Read the model definition and answer for the solid it produces. Units are mm, in the model's axes. A direction names the side the tool comes from. Coordinates: 2 decimals unless noted, no trailing zeros. Order: outer loops, then holes, each group sorted by start corner. A loop starts at its lowest first (then second) coordinate and runs counter-clockwise, first axis right, second up. Notation, with made-up numbers: (-19, 10) -> (36, 10) arc R17 ccw to (36, 38) -> close; hole circle Ø1 at (-33.75, 33). An arc over 180 degrees is marked (long way). Answer as a JSON object with one key per item and string values. Group by question number.
1) A tool of negligible diameter and unlimited length cuts with its end or side. For faces 1 (the flat face through (-1, -1, -2)), 2 (the flat face through (18, 33, 128)), 3 (the flat face through (95, -4, -120)), 4 (the flat face through (100.08, -9.04, -1.68)), from which of +Z, -Z, +X, -X, +Y, -Y can it reach the whole face along a straight path? Write none if from no direction.
2) Section D-D on z = -28.5 is taken. Determine the outline of the cut face in (x, y).
3) Consider L1, parallel to X at y = -0.4, z = -52; L2, parallel to Y at x = -5.5, z = 36; L3, parallel to Z at x = -0.5, y = 13.5. Determine where each line is inside the solid, lowest interval first.
4) Section B-B on x = 0 is taken. Determine the outline of the cut face in (y, z).
5) Section C-C on y = 63.5 is taken. Determine the outline of the cut face in (x, z).
6) Given pin 1 (9 mm diameter, centred on x = 93.5, y = -6, fed in from +Z); pin 2 (19.5 mm diameter, centred on y = -12.5, z = -134, fed in from +X); pin 3 (1 mm diameter, centred on y = 0, z = -43.5, fed in from +X), each flat-ended and moving along its own axis, determine where each tip first touches the part or whether it passes through.
7) Determine the mould class of faces 5 (the flat face through (95, -4, 120)), 6 (the flat face through (-95.674, -3.727, 1.68)), 7 (the flat face through (-95, -4, -120)), 8 (the cylindrical face through (0.88, -0.49, -114.98)) for opening direction Z: released by +Z, released by -Z, zero draft, split by the parting line, or undercut.
8) Section A-A on z = -111 is taken. Determine the outline of the cut face in (x, y), and give its area (3 significant figures).
from build123d import *

# Parameters (mm, degrees)
ESBO_O1_W                 = 180
ESBO_O1_H                 = 250
FLANGE_BASE1_DEPTH        = 1
ESBO_O6_R                 = 2.4
ESBO_O6_R_2               = 20
CORTE_EXTRUS_O1_DEPTH     = 10
FILETE1_R                 = 5
ARESTA_FLANGE1_DEPTH      = 170
ARESTA_FLANGE2_DEPTH      = 240
ARESTA_FLANGE2_BEND_DEPTH = 240
FILETE2_R                 = 5
ARESTA_FLANGE3_DEPTH      = 170
FILETE3_R                 = 70
ESBO_O29_W                = 23
ESBO_O29_H                = 57
CORTE_EXTRUS_O2_DEPTH     = 308.427518565
FILETE4_R                 = 2
CORTE_EXTRUS_O3_REACH     = 220.213
ESBO_O32_R                = 2.4


# Sheet-metal steps are written as plain solids
with BuildPart() as part:
    # Esbo_o1 → Flange-base1 (new body)
    with BuildSketch(Plane(origin=(0, 0, 0), x_dir=(1, 0, 0), z_dir=(0, 1, 0))):
        Rectangle(ESBO_O1_W, ESBO_O1_H)
    extrude(amount=-FLANGE_BASE1_DEPTH)

    # Esbo_o6 → Corte-extrus_o1 (cut)
    with BuildSketch(Plane(origin=(0, 0, 0), x_dir=(1, 0, 0), z_dir=(0, 1, 0))):
        with Locations(Location((-25, 52, 0), (0, 0, 270))):
            Circle(ESBO_O6_R)
        with Locations(Location((25, 52, 0), (0, 0, 270))):
            Circle(ESBO_O6_R)
        with Locations(Location((-25, -40, 0), (0, 0, 270))):
            Circle(ESBO_O6_R)
        with Locations(Location((25, -40, 0), (0, 0, 270))):
            Circle(ESBO_O6_R)
        with Locations(Location((-25, -46, 0), (0, 0, 270))):
            Circle(ESBO_O6_R)
        with Locations(Location((25, -46, 0), (0, 0, 270))):
            Circle(ESBO_O6_R)
        with Locations(Location((-25, 46, 0), (0, 0, 270))):
            Circle(ESBO_O6_R)
        with Locations(Location((25, 46, 0), (0, 0, 270))):
            Circle(ESBO_O6_R)
        with Locations(Location((-25, 58, 0), (0, 0, 270))):
            Circle(ESBO_O6_R)
        with Locations(Location((25, 58, 0), (0, 0, 270))):
            Circle(ESBO_O6_R)
        with Locations(Location((-25, -34, 0), (0, 0, 270))):
            Circle(ESBO_O6_R)
        with Locations(Location((25, -34, 0), (0, 0, 270))):
            Circle(ESBO_O6_R)
        with Locations(Location((-25, 40, 0), (0, 0, 270))):
            Circle(ESBO_O6_R)
        with Locations(Location((25, 40, 0), (0, 0, 270))):
            Circle(ESBO_O6_R)
        with Locations(Location((-25, -52, 0), (0, 0, 270))):
            Circle(ESBO_O6_R)
        with Locations(Location((25, -52, 0), (0, 0, 270))):
            Circle(ESBO_O6_R)
        with Locations(Location((-25, 34, 0), (0, 0, 270))):
            Circle(ESBO_O6_R)
        with Locations(Location((25, 34, 0), (0, 0, 270))):
            Circle(ESBO_O6_R)
        with Locations(Location((-25, -58, 0), (0, 0, 270))):
            Circle(ESBO_O6_R)
        with Locations(Location((25, -58, 0), (0, 0, 270))):
            Circle(ESBO_O6_R)
        with Locations(Location((0, 95, 0), (0, 0, 270))):
            Circle(ESBO_O6_R_2)
    extrude(amount=-CORTE_EXTRUS_O1_DEPTH, mode=Mode.SUBTRACT)

    # Filete1
    filete1_edges = [part.edges().sort_by_distance(p)[0] for p in [
        (90, -0.5, 125),
        (-90, -0.5, 125),
        (-90, -0.5, -125),
        (90, -0.5, -125),
    ]]
    fillet(filete1_edges, radius=FILETE1_R)

    # Aresta-Flange1 section (across the edge) → Aresta-Flange1 (add)
    with BuildSketch(Plane(origin=(-85, -1, -126.151592105), x_dir=(0, -0.7431448254773979, 0.6691306063588541), z_dir=(1, 0, 0))):
        with BuildLine():
            Line((-1, 1.151592105), (-1, 30))
            Line((-1, 30), (0, 30))
            Line((0, 30), (0, 1.151592105))
            ThreePointArc((0, 1.151592105), (0.199258721, 0.076488256), (0.770565524, -0.855799714))
            Line((0.770565524, -0.855799714), (0.027420698, -1.52493032))
            ThreePointArc((0.027420698, -1.52493032), (-0.734321706, -0.281879693), (-1, 1.151592105))
        make_face()
    extrude(amount=ARESTA_FLANGE1_DEPTH)

    # Aresta-Flange2 section (across the edge) → Aresta-Flange2 (add)
    with BuildSketch(Plane(origin=(91.151592105, -1, -120), x_dir=(-0.6691306063588541, -0.7431448254773979, 0), z_dir=(0, 0, 1))):
        with BuildLine():
            Line((-1, 1.151592105), (-1, 16.05))
            Line((-1, 16.05), (0, 16.05))
            Line((0, 16.05), (0, 1.151592105))
            ThreePointArc((0, 1.151592105), (0.199258721, 0.076488256), (0.770565524, -0.855799714))
            Line((0.770565524, -0.855799714), (0.027420698, -1.52493032))
            ThreePointArc((0.027420698, -1.52493032), (-0.734321706, -0.281879693), (-1, 1.151592105))
        make_face()
    extrude(amount=ARESTA_FLANGE2_DEPTH)

    # Aresta-Flange2 section 2 (across the edge) → Aresta-Flange2 bend (add)
    with BuildSketch(Plane(origin=(-91.151592105, -1, 120), x_dir=(0.6691306063588541, -0.7431448254773979, 0), z_dir=(0, 0, -1))):
        with BuildLine():
            Line((-1, 1.151592105), (-1, 16.05))
            Line((-1, 16.05), (0, 16.05))
            Line((0, 16.05), (0, 1.151592105))
            ThreePointArc((0, 1.151592105), (0.199258721, 0.076488256), (0.770565524, -0.855799714))
            Line((0.770565524, -0.855799714), (0.027420698, -1.52493032))
            ThreePointArc((0.027420698, -1.52493032), (-0.734321706, -0.281879693), (-1, 1.151592105))
        make_face()
    extrude(amount=ARESTA_FLANGE2_BEND_DEPTH)

    # Filete2
    filete2_edges = [part.edges().sort_by_distance(p)[0] for p in [
        (-85, -20.702345778, -148.780502173),
        (85, -20.702345778, -148.780502173),
        (103.413631857, -11.367973819, -120),
        (103.413631857, -11.367973819, 120),
        (-103.413631857, -11.367973819, 120),
        (-103.413631857, -11.367973819, -120),
    ]]
    fillet(filete2_edges, radius=FILETE2_R)

    # Aresta-Flange3 section (across the edge) → Aresta-Flange3 (add)
    with BuildSketch(Plane(origin=(-85, 0, 128), x_dir=(0, 0, -1), z_dir=(1, 0, 0))):
        with BuildLine():
            Line((-1, 3), (-1, 80))
            Line((-1, 80), (0, 80))
            Line((0, 80), (0, 3))
            ThreePointArc((0, 3), (0.878679656, 0.878679656), (3, 0))
            Line((3, 0), (3, -1))
            ThreePointArc((3, -1), (0.171572875, 0.171572875), (-1, 3))
        make_face()
    extrude(amount=ARESTA_FLANGE3_DEPTH)

    # Filete3
    filete3_edges = [part.edges().sort_by_distance(p)[0] for p in [
        (-85, 80, 128.5),
        (85, 80, 128.5),
    ]]
    fillet(filete3_edges, radius=FILETE3_R)

    # Esbo_o29 → Corte-extrus_o2 (cut, through all)
    with BuildSketch(Plane.XY.offset(129)):
        with Locations((0, 51.5)):
            Rectangle(ESBO_O29_W, ESBO_O29_H)
    extrude(amount=-CORTE_EXTRUS_O2_DEPTH, mode=Mode.SUBTRACT)

    # Filete4
    filete4_edges = [part.edges().sort_by_distance(p)[0] for p in [
        (-11.5, 80, 128.5),
        (11.5, 80, 128.5),
        (11.5, 23, 128.5),
        (-11.5, 23, 128.5),
    ]]
    fillet(filete4_edges, radius=FILETE4_R)

    # Esbo_o32 → Corte-extrus_o3 (cut, up to next)
    with BuildSketch(Plane(origin=(40.983697788, 45.517007667, 0), x_dir=(0.7431448254773984, -0.6691306063588536, 0), z_dir=(0.6691306063588536, 0.7431448254773984, 0)), mode=Mode.PRIVATE) as corte_extrus_o3_sk1:
        with Locations(Location((77.008760666, 0, 0), (0, 0, 180))):
            Circle(ESBO_O32_R)
    corte_extrus_o3_tool1 = extrude(corte_extrus_o3_sk1.sketch, amount=-CORTE_EXTRUS_O3_REACH, mode=Mode.PRIVATE) & part.part
    # Esbo_o32 → Corte-extrus_o3 (cut, up to next)
    with BuildSketch(Plane(origin=(40.983697788, 45.517007667, 0), x_dir=(0.7431448254773984, -0.6691306063588536, 0), z_dir=(0.6691306063588536, 0.7431448254773984, 0)), mode=Mode.PRIVATE) as corte_extrus_o3_sk2:
        with Locations(Location((77.008760666, -100, 0), (0, 0, 180))):
            Circle(ESBO_O32_R)
    corte_extrus_o3_tool2 = extrude(corte_extrus_o3_sk2.sketch, amount=-CORTE_EXTRUS_O3_REACH, mode=Mode.PRIVATE) & part.part
    # Esbo_o32 → Corte-extrus_o3 (cut, up to next)
    with BuildSketch(Plane(origin=(40.983697788, 45.517007667, 0), x_dir=(0.7431448254773984, -0.6691306063588536, 0), z_dir=(0.6691306063588536, 0.7431448254773984, 0)), mode=Mode.PRIVATE) as corte_extrus_o3_sk3:
        with Locations(Location((77.008760666, -50, 0), (0, 0, 180))):
            Circle(ESBO_O32_R)
    corte_extrus_o3_tool3 = extrude(corte_extrus_o3_sk3.sketch, amount=-CORTE_EXTRUS_O3_REACH, mode=Mode.PRIVATE) & part.part
    # Esbo_o32 → Corte-extrus_o3 (cut, up to next)
    with BuildSketch(Plane(origin=(40.983697788, 45.517007667, 0), x_dir=(0.7431448254773984, -0.6691306063588536, 0), z_dir=(0.6691306063588536, 0.7431448254773984, 0)), mode=Mode.PRIVATE) as corte_extrus_o3_sk4:
        with Locations(Location((77.008760666, 50, 0), (0, 0, 180))):
            Circle(ESBO_O32_R)
    corte_extrus_o3_tool4 = extrude(corte_extrus_o3_sk4.sketch, amount=-CORTE_EXTRUS_O3_REACH, mode=Mode.PRIVATE) & part.part
    # Esbo_o32 → Corte-extrus_o3 (cut, up to next)
    with BuildSketch(Plane(origin=(40.983697788, 45.517007667, 0), x_dir=(0.7431448254773984, -0.6691306063588536, 0), z_dir=(0.6691306063588536, 0.7431448254773984, 0)), mode=Mode.PRIVATE) as corte_extrus_o3_sk5:
        with Locations(Location((77.008760666, 100, 0), (0, 0, 180))):
            Circle(ESBO_O32_R)
    corte_extrus_o3_tool5 = extrude(corte_extrus_o3_sk5.sketch, amount=-CORTE_EXTRUS_O3_REACH, mode=Mode.PRIVATE) & part.part
    corte_extrus_o3_1 = corte_extrus_o3_tool1.solids().sort_by_distance((98.21236, -6.011911, 0))[0]
    add(corte_extrus_o3_1, mode=Mode.SUBTRACT)
    corte_extrus_o3_2 = corte_extrus_o3_tool2.solids().sort_by_distance((98.21236, -6.011911, 100))[0]
    add(corte_extrus_o3_2, mode=Mode.SUBTRACT)
    corte_extrus_o3_3 = corte_extrus_o3_tool3.solids().sort_by_distance((98.21236, -6.011911, 50))[0]
    add(corte_extrus_o3_3, mode=Mode.SUBTRACT)
    corte_extrus_o3_4 = corte_extrus_o3_tool4.solids().sort_by_distance((98.21236, -6.011911, -50))[0]
    add(corte_extrus_o3_4, mode=Mode.SUBTRACT)
    corte_extrus_o3_5 = corte_extrus_o3_tool5.solids().sort_by_distance((98.21236, -6.011911, -100))[0]
    add(corte_extrus_o3_5, mode=Mode.SUBTRACT)
    corte_extrus_o3 = corte_extrus_o3_1 + corte_extrus_o3_2 + corte_extrus_o3_3 + corte_extrus_o3_4 + corte_extrus_o3_5  # Corte-extrus_o3 as one shape, for the pattern or mirror that repeats it

    # Espelhar1: Corte-extrus_o3 across plane
    add(corte_extrus_o3.mirror(Plane(origin=(0, 0, 0), x_dir=(0, 0, 1), z_dir=(1, 0, 0))), mode=Mode.SUBTRACT)


solid = part.part
Worked answers:
{
 "1": {"face 1": "+Z, -Y", "face 2": "-Z, +X, -X, +Y", "face 3": "-Z, +X, +Y, -Y", "face 4": "+Z, -Z, -Y"},
 "2": {"outline": "(-103.75, -11) -> (-103.08, -11.74) -> (-92.01, -1.77) arc R3 cw to (-90, -1) -> (90, -1) arc R3 cw to (92.01, -1.77) -> (103.08, -11.74) -> (103.75, -11) -> (92.68, -1.03) arc R4 ccw to (90, 0) -> (-90, 0) arc R4 ccw to (-92.68, -1.03) -> close"},
 "3": {"L1": "x = -91.74 to -27.4, -22.6 to 22.6, 27.4 to 91.74", "L2": "y = -1 to 0", "L3": "z = 128 to 129"},
 "4": {"outline": "(-21.07, -148.45) -> (-20.33, -149.12) -> (-1.03, -127.68) arc R4 ccw to (0, -125) -> (0, -115) -> (-1, -115) -> (-1, -125) arc R3 cw to (-1.77, -127.01) -> close; (-1, -75) -> (0, -75) -> (0, 125) arc R3 cw to (3, 128) -> (23, 128) -> (23, 129) -> (3, 129) arc R4 ccw to (-1, 125) -> close"},
 "5": {"outline": "(-60.14, 128) -> (-11.5, 128) -> (-11.5, 129) -> (-60.14, 129) -> close; (11.5, 128) -> (60.14, 128) -> (60.14, 129) -> (11.5, 129) -> close"},
 "6": {"pin 1": "stops at z = 120", "pin 2": "stops at x = 85", "pin 3": "stops at x = 91.94"},
 "7": {"face 5": "released by +Z", "face 6": "zero draft", "face 7": "released by -Z", "face 8": "undercut"},
 "8": {"outline": "(-103.75, -11) -> (-103.08, -11.74) -> (-92.01, -1.77) arc R3 cw to (-90, -1) -> (-12, -1) -> (-12, 0) -> (-90, 0) arc R4 ccw to (-92.68, -1.03) -> close; (12, -1) -> (90, -1) arc R3 cw to (92.01, -1.77) -> (103.08, -11.74) -> (103.75, -11) -> (92.68, -1.03) arc R4 ccw to (90, 0) -> (12, 0) -> close", "area": "191 mm²"}
}
